Input: dimensioned drawing with shaded views. Units: mm. Origin: part minimum x, y, z. A direction names the side the tool comes from. Coordinates: 2 decimals unless noted, no trailing zeros. Loops run counter-clockwise (first coordinate to the right, second up) from the corner with the lowest first, then second, coordinate; pieces in that order, holes last.
Item 1: Contact query for flat-ended pins moving along their axis: P1, Ø2, axis at y = 2, z = 11, coming from the +X side; P2, Ø3, axis at x = 25, y = 5, coming from the +Z side; P3, Ø5, axis at x = 15, z = 10, coming from the -Y side; P4, Ø3, axis at x = 4, y = 5, coming from the +Z side. Output: stop coordinate, or through.
Item 2: Reachability of the marked faces 1, 2, 3, 4 and 5 from +Z, -Z, +X, -X, +Y, -Y: full face, straight path, thin tool, end or side. Return the list, or none.
Item 3: Ray query, line 1 along Z through (x, y) = (15, 6.95); line 2 along X through (y, z) = (4.25, 11.5); line 3 along Y through (x, z) = (25, 1.5). Return the intervals inside material, ascending.
Item 4: Section D-D on y = 3.5. Return loops of the section in (x, z), and give its area (3 significant figures).
Item 5: Pull-direction query (X, two-part tool) for the marked faces 6, 7, 8 and 9; classes: released by +X, released by -X, zero draft, split by the parting line, or undercut.
Item 6: Section A-A on z = 10. Return loops of the section in (x, y).
Item 7: Section B-B on x = 5. Return loops of the section in (y, z), and give its area (3 significant figures).
Item 8: Section C-C on y = 1.5. Return loops of the section in (x, z), and give its area (3 significant figures).
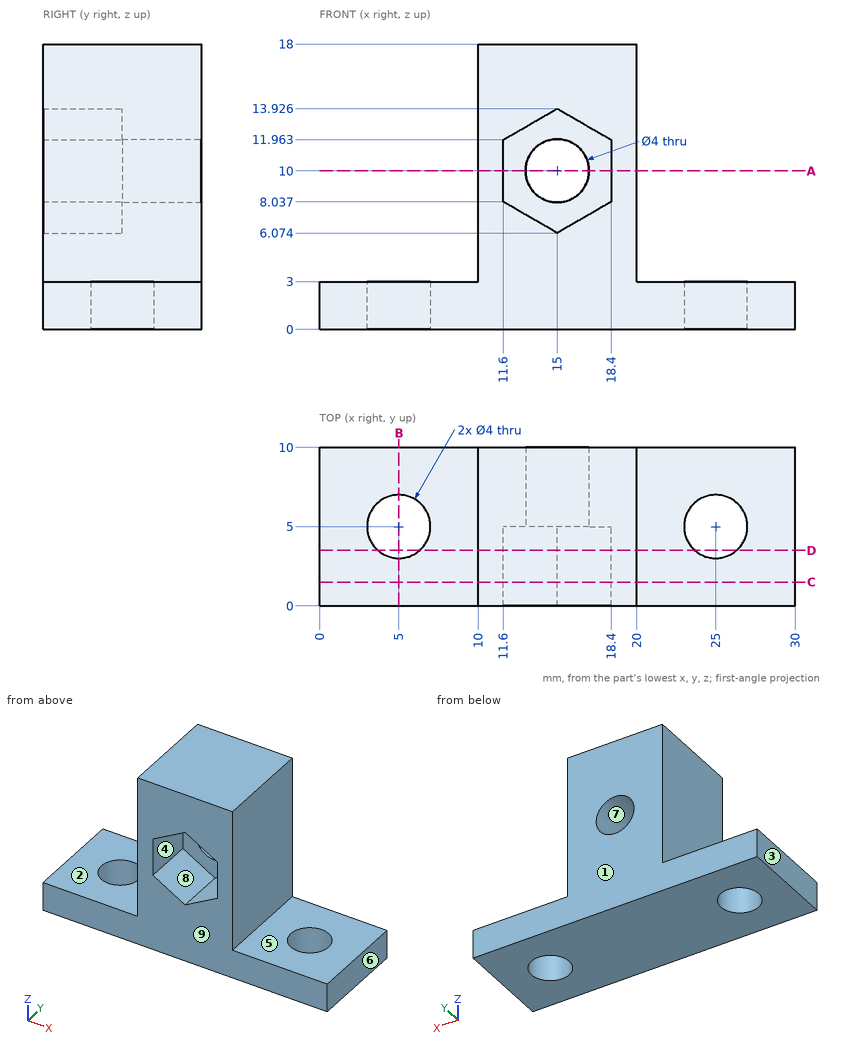
Results found:
1. P1: stops at x = 20
1. P2: passes through
1. P3: stops at y = 5
1. P4: stops at z = 3
2. face 1: +Z, -Z, +X, -X, +Y
2. face 2: +Z, -X, +Y, -Y
2. face 3: +Z, -Z, -X, +Y, -Y
2. face 4: -Y
2. face 5: +Z, +X, +Y, -Y
3. line 1: z = 0 to 8, 12 to 18
3. line 2: x = 10 to 11.6, 18.4 to 20
3. line 3: y = 0 to 3, 7 to 10
4. outline: (0, 0) - (3.68, 0) - (3.68, 3) - (0, 3) - close; (6.32, 0) - (23.68, 0) - (23.68, 3) - (20, 3) - (20, 18) - (10, 18) - (10, 3) - (6.32, 3) - close; (26.32, 0) - (30, 0) - (30, 3) - (26.32, 3) - close; hole (11.6, 8.04) - (15, 6.07) - (18.4, 8.04) - (18.4, 11.96) - (15, 13.93) - (11.6, 11.96) - close
4. area: 184 mm2
5. face 6: released by +X
5. face 7: undercut
5. face 8: undercut
5. face 9: zero draft
6. outline: (10, 0) - (11.6, 0) - (11.6, 5) - (13, 5) - (13, 10) - (10, 10) - close; (17, 5) - (18.4, 5) - (18.4, 0) - (20, 0) - (20, 10) - (17, 10) - close
7. outline: (0, 0) - (3, 0) - (3, 3) - (0, 3) - close; (7, 0) - (10, 0) - (10, 3) - (7, 3) - close
7. area: 18.0 mm2
8. outline: (0, 0) - (30, 0) - (30, 3) - (20, 3) - (20, 18) - (10, 18) - (10, 3) - (0, 3) - close; hole (11.6, 8.04) - (15, 6.07) - (18.4, 8.04) - (18.4, 11.96) - (15, 13.93) - (11.6, 11.96) - close
8. area: 200 mm2
